Work out the finished part from the listing and answer in its coordinate system (mm). A direction names the side the tool comes from. Coordinates: 2 decimals unless noted, no trailing zeros. Loops run counter-clockwise (first coordinate to the right, second up) from the corner with the lowest first, then second, coordinate; pieces in that order, holes last. Notation, with made-up numbers: (78, 0) - (102, 0) arc R27 ccw to (102, 31) - close; hole circle Ø10 at (-9.75, 49). An arc over 180 degrees is marked (long way). Write each question's results on one line, items separated by ' | '. Start each with the question number.
1. Determine the mould class of faces 6 (the flat face through (42, 0, 12)), 7 (the flat face through (28, 8, 20.226)), 8 (the flat face through (66, 6, 11.644)), 9 (the flat face through (42, 17, 0)) for opening direction Z: released by +Z, released by -Z, zero draft, split by the parting line, or undercut.
2. A cutting plane is placed at B-B on y = 6. Determine the outline of the cut face in (x, z).
3. A cutting plane is placed at D-D on x = 66.5. Determine the outline of the cut face in (y, z), then the cut area to 3 significant figures.
4. This flat-tipped pin is pushed along its axis until it touches: P1, Ø1.5, axis at x = 31.5, z = 25, coming from the +Y side. Where does it stop, or does it pass through?
5. Which of the six approach directions +Z, -Z, +X, -X, +Y, -Y give full straight-line access (tool end or side, diameter ignored) to faces 1 (the flat face through (56.557, 4.268, 26.915)), 2 (the flat face through (41.85, 6, 22)), 3 (the flat face through (60.858, 4, 8)), 4 (the flat face through (70.858, 25, 15)), 5 (the flat face through (13.85, 25, 15))?
6. A cutting plane is placed at A-A on x = 33.5. Determine the outline of the cut face in (y, z).
7. Find the intervals of material crossed by line 1 along Z through (x, y) = (60.5, 6); line 2 along Z through (x, y) = (18, 5); line 3 along Y through (x, z) = (52, 2.5), in increasing order. Write a range as [from, to].
8. A cutting plane is placed at C-C on z = 4.75. Determine the outline of the cut face in (x, y).
from build123d import *

# Parameters (mm, degrees)
SKETCH_1_W          = 57.008230548
SKETCH_1_H          = 50.142083818
EXTRUDE_2_DEPTH     = 30
CUT_EXTRUDE_1_DEPTH = 82.634348897
CUT_EXTRUDE_2_DEPTH = 10
CUT_EXTRUDE_3_DEPTH = 28
CUT_EXTRUDE_4_DEPTH = 82.634348897


with BuildPart() as part:
    # 草圖1 → 填料-伸長2 (new body)
    with BuildSketch(Plane.XY):
        with Locations((42.353664605, 25.071041909)):
            Rectangle(SKETCH_1_W, SKETCH_1_H)
    extrude(amount=EXTRUDE_2_DEPTH)

    # 草圖2 → 除料-伸長1 (cut, through all)
    with BuildSketch(Plane.ZY.offset(-13.849549331)):
        Polygon((30, 50.142083818), (0, 33.426531832), (0, 50.142083818), align=None)
    extrude(amount=-CUT_EXTRUDE_1_DEPTH, mode=Mode.SUBTRACT)

    # 草圖3 → 除料-伸長2 (cut)
    with BuildSketch(Plane(origin=(70.857779879, 0, 0), x_dir=(0, 0, -1), z_dir=(1, 0, 0))):
        Polygon((-11.643819947, 12.450406502), (-11.643819947, 0), (0, 0), align=None)
    extrude(amount=-CUT_EXTRUDE_2_DEPTH, mode=Mode.SUBTRACT)

    # 草圖6 → 除料-伸長3 (cut)
    with BuildSketch(Plane.ZY.offset(-13.849549331)):
        Polygon((30, 0), (20.225842112, 16.602142494), (20.225842112, 0), align=None)
    extrude(amount=-CUT_EXTRUDE_3_DEPTH, mode=Mode.SUBTRACT)

    # 草圖7 → 除料-伸長4 (cut, through all)
    with BuildSketch(Plane(origin=(70.857779879, 0, 0), x_dir=(0, 0, -1), z_dir=(1, 0, 0))):
        Polygon((-30, 0), (-23.742805889, 8.65630368), (-23.742805889, 0), align=None)
    extrude(amount=-CUT_EXTRUDE_4_DEPTH, mode=Mode.SUBTRACT)


solid = part.part
Values:
1) face 6: zero draft | face 7: undercut | face 8: undercut | face 9: released by -Z
2) outline: (13.85, 0) - (70.86, 0) - (70.86, 5.61) - (60.86, 5.61) - (60.86, 11.64) - (70.86, 11.64) - (70.86, 23.74) - (41.85, 23.74) - (41.85, 20.23) - (13.85, 20.23) - close; (13.85, 26.47) - (41.85, 26.47) - (41.85, 25.66) - (70.86, 25.66) - (70.86, 30) - (13.85, 30) - close
3) outline: (0, 0) - (33.43, 0) - (50.14, 30) - (0, 30) - (8.66, 23.74) - (0, 23.74) - (0, 11.64) - (12.45, 11.64) - close | area: 1,150 mm^2
4) P1: y = 47.77
5) face 1: +X, -X, -Y | face 2: -X, -Y | face 3: +X, -Y | face 4: +Z, -Z, +X, +Y, -Y | face 5: +Z, -Z, -X, +Y, -Y
6) outline: (0, 0) - (33.43, 0) - (50.14, 30) - (0, 30) - (16.6, 20.23) - (0, 20.23) - close
7) line 1: [0, 23.74], [25.66, 30] | line 2: [0, 20.23], [27.06, 30] | line 3: [0, 34.82]
8) outline: (13.85, 0) - (60.86, 0) - (60.86, 5.08) - (70.86, 5.08) - (70.86, 36.07) - (13.85, 36.07) - close
